Part model, mm, in its own coordinate system. Face numbers are marked on the shaded views. A direction names the side the tool comes from. Give positions to 0.01 mm unless a question says otherwise; leave off trailing zeros. Order: outer loops, then holes, each group sorted by start corner. A loop starts at its lowest first (then second) coordinate and runs counter-clockwise, first axis right, second up. Notation, with made-up numbers: M 32.25,20.25 L 51.25,20.25 A32 cw 51.25,56.25 Z; hole C 64,61.5 d8. An arc over 180 degrees is marked long. Return JSON: item names as keys, results as strings.
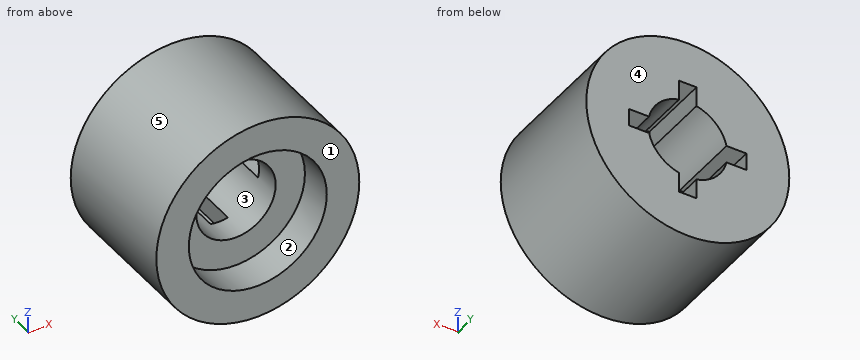
from build123d import *

# Parameters (mm, degrees)
F0_R     = 4.09
F0_R_2   = 1.6
F1_DEPTH = 5.45
F2_R     = 2.78
F3_DEPTH = 1.39
F5_DEPTH = 3


with BuildPart() as f1:
    # F0 (on Front) → F1 (new body)
    with BuildSketch(Plane.XZ):
        Circle(F0_R)
        Circle(F0_R_2, mode=Mode.SUBTRACT)
    extrude(amount=F1_DEPTH)

    # F2 (on face) → F3 (cut)
    with BuildSketch(Plane.XZ.offset(5.45)):
        Circle(F2_R)
    extrude(amount=-F3_DEPTH, mode=Mode.SUBTRACT)

    # F4 (on face) → F5 (cut)
    with BuildSketch(Plane(origin=(0, 0, 0), x_dir=(-1, 0, 0), z_dir=(0, 1, 0))):
        with BuildLine():
            Line((-0.35, 2.3612494996), (-0.35, 1.5612494996))
            ThreePointArc((-0.35, 1.5612494996), (0, 1.6), (0.35, 1.5612494996))
            Line((0.35, 1.5612494996), (0.35, 2.3612494996))
            Line((0.35, 2.3612494996), (-0.35, 2.3612494996))
        make_face()
        with BuildLine():
            Line((2.3612494996, 0.35), (1.5612494996, 0.35))
            ThreePointArc((1.5612494996, 0.35), (1.5902828678, 0.1760693054), (1.6, 0))
            ThreePointArc((1.6, 0), (1.5902828678, -0.1760693054), (1.5612494996, -0.35))
            Line((1.5612494996, -0.35), (2.3612494996, -0.35))
            Line((2.3612494996, -0.35), (2.3612494996, 0.35))
        make_face()
        with BuildLine():
            ThreePointArc((0.35, -1.5612494996), (0, -1.6), (-0.35, -1.5612494996))
            Line((-0.35, -1.5612494996), (-0.35, -2.3612494996))
            Line((-0.35, -2.3612494996), (0.35, -2.3612494996))
            Line((0.35, -2.3612494996), (0.35, -1.5612494996))
        make_face()
        with BuildLine():
            ThreePointArc((-1.5612494996, -0.35), (-1.6, 0), (-1.5612494996, 0.35))
            Line((-1.5612494996, 0.35), (-2.3612494996, 0.35))
            Line((-2.3612494996, 0.35), (-2.3612494996, -0.35))
            Line((-2.3612494996, -0.35), (-1.5612494996, -0.35))
        make_face()
    extrude(amount=-F5_DEPTH, mode=Mode.SUBTRACT)


solid = f1.part
Q1. Probe line 1 along Z through (x, y) = (0, -4.8); line 2 along Z through (x, y) = (0, -1.15); line 3 along Y through (x, z) = (-1.75, 1.25). List the from-to ranges inside material, lowest first.
Established:
{"line 1": "z = -4.09 to -2.78, 2.78 to 4.09", "line 2": "z = -4.09 to -2.36, 2.36 to 4.09", "line 3": "y = -4.06 to 0"}
Q2. Band-saw the part on B-B (y = -2.5). Give the cut face in (x, z), then the cut area to 3 significant figures.
Established:
{"outline": "C 0,0 d8.18; hole M -2.36,-0.35 L -1.56,-0.35 A1.6 ccw -0.35,-1.56 L -0.35,-2.36 L 0.35,-2.36 L 0.35,-1.56 A1.6 ccw 1.56,-0.35 L 2.36,-0.35 L 2.36,0.35 L 1.56,0.35 A1.6 ccw 0.35,1.56 L 0.35,2.36 L -0.35,2.36 L -0.35,1.56 A1.6 ccw -1.56,0.35 L -2.36,0.35 Z", "area": "42.3 mm²"}
Q3. Two-plate mould, pull along Z, no slides. Class the marked faces 3, 4 and 5: +Z half, -Z half, draft (parallel to the pull), parting line (faces both ways), or undercut.
Established:
{"face 3": "undercut", "face 4": "draft", "face 5": "parting line"}
Q4. Band-saw the part on D-D (z = -2.5). Give the cut face in (x, y), then the cut area to 3 significant figures.
Established:
{"outline": "M -3.24,-5.45 L -1.22,-5.45 L -1.22,-4.06 L 1.22,-4.06 L 1.22,-5.45 L 3.24,-5.45 L 3.24,0 L -3.24,0 Z", "area": "31.9 mm²"}
Q5. Pin check, flat tips, straight feed: pin 1 (1.5 mm diameter, centred on y = -2, z = 3, fed in from +X); pin 2 (0.6 mm diameter, centred on x = -2, y = -1.5, fed in from +Z); pin 3 (0.6 mm diameter, centred on y = -1.5, z = -2, fed in from -X). Stop position of each tip, or through.
Established:
{"pin 1": "stops at x = 3.42", "pin 2": "stops at z = 3.72", "pin 3": "stops at x = -3.72"}
Q6. 3-axis set-ups, long thin cutter, end or side, ignore diameter. For the marked faces 1 and 2: which of +Z, -Z, +X, -X, +Y, -Y reach the whole face in a straight line?
Established:
{"face 1": "+Z, -Z, +X, -X, -Y", "face 2": "-Y"}
Q7. Band-saw the part on C-C (z = 0). Give the cut face in (x, y), then the cut area to 3 significant figures.
Established:
{"outline": "M -4.09,-5.45 L -2.78,-5.45 L -2.78,-4.06 L -1.6,-4.06 L -1.6,-3 L -2.36,-3 L -2.36,0 L -4.09,0 Z; M 1.6,-4.06 L 2.78,-4.06 L 2.78,-5.45 L 4.09,-5.45 L 4.09,0 L 2.36,0 L 2.36,-3 L 1.6,-3 Z", "area": "19.3 mm²"}
Q8. Band-saw the part on A-A (x = 0). Give the cut face in (y, z).
Established:
{"outline": "M -5.45,-4.09 L 0,-4.09 L 0,-2.36 L -3,-2.36 L -3,-1.6 L -4.06,-1.6 L -4.06,-2.78 L -5.45,-2.78 Z; M -5.45,2.78 L -4.06,2.78 L -4.06,1.6 L -3,1.6 L -3,2.36 L 0,2.36 L 0,4.09 L -5.45,4.09 Z"}
